```python
from build123d import *

# Parameters (mm, degrees)
F1_DEPTH = 25
F0_W     = 25
F0_H     = 3
F0_H_2   = 15
F2_DEPTH = 3
F3_R     = 2
F4_DEPTH = 25
F3_R_2   = 5
F5_DEPTH = 10


with BuildPart() as f1:
    # F0 (on Top) → F1 (new body)
    with BuildSketch(Plane.XY):
        with BuildLine():
            ThreePointArc((-51.955607151, 33.064927277), (-39.2002565409, 19.8557934078), (-21.4914605021, 15))
            Line((-21.4914605021, 15), (3.5085394979, 15))
            ThreePointArc((3.5085394979, 15), (21.2173355366, 19.8557934078), (33.9726861467, 33.064927277))
            Line((33.9726861467, 33.064927277), (31.3403677316, 34.5039893887))
            ThreePointArc((31.3403677316, 34.5039893887), (19.687169914, 22.4362184053), (3.5085394979, 18))
            Line((3.5085394979, 18), (-21.4914605021, 18))
            ThreePointArc((-21.4914605021, 18), (-37.6700909183, 22.4362184053), (-49.3232887359, 34.5039893887))
            Line((-49.3232887359, 34.5039893887), (-51.955607151, 33.064927277))
        make_face()
    extrude(amount=F1_DEPTH)



with BuildPart() as f1b:
    # F0 (on Top) → F1, piece 2 (new body)
    with BuildSketch(Plane.XY):
        with Locations((-8.9914605021, -1.5)):
            Rectangle(F0_W, F0_H)
    extrude(amount=F1_DEPTH)


with BuildPart() as f1_1:
    add(f1.part)

    add(f1b.part)  # F2 merges F1b
    # F0 (on Top) → F2 (join)
    with BuildSketch(Plane.XY):
        with Locations((-8.9914605021, 7.5)):
            Rectangle(F0_W, F0_H_2)
    extrude(amount=F2_DEPTH)

    # F3 (on face) → F4 (cut)
    with BuildSketch(Plane(origin=(0, 18, 0), x_dir=(-1, 0, 0), z_dir=(0, 1, 0))):
        with Locations((15.4914605021, 12.5)):
            Circle(F3_R)
        with Locations((2.4914605021, 12.5)):
            Circle(F3_R)
    extrude(amount=-F4_DEPTH, mode=Mode.SUBTRACT)

    # F3 (on face) → F5 (cut)
    with BuildSketch(Plane(origin=(0, 18, 0), x_dir=(-1, 0, 0), z_dir=(0, 1, 0))):
        with Locations((15.4914605021, 12.5)):
            Circle(F3_R_2)
        with Locations((15.4914605021, 12.5)):
            Circle(F3_R, mode=Mode.SUBTRACT)
        with Locations((2.4914605021, 12.5)):
            Circle(F3_R_2)
        with Locations((2.4914605021, 12.5)):
            Circle(F3_R, mode=Mode.SUBTRACT)
    extrude(amount=-F5_DEPTH, mode=Mode.SUBTRACT)


solid = f1_1.part
```
The model under review builds one solid part; all positions refer to its coordinate system, in mm. A direction names the side the tool comes from. Coordinates: 2 decimals unless noted, no trailing zeros. Write each loop counter-clockwise with the first axis right and the second up, starting at its lowest first coordinate (ties: lowest second). Pieces come first, ordered by that corner, then holes. Notation, with made-up numbers: (68.5, 12) - (74.5, 12) arc R17 cw to (74.5, 16) - close; hole circle Ø9 at (69, -28). An arc over 180 degrees is marked (long way). Write item = value, one per line.
(1) Consider section C-C, the plane z = 19.25. Give the boundary of the cut face in (x, y).
Result sheet:
outline = (-51.96, 33.06) arc R34.72 ccw to (-21.49, 15) - (3.51, 15) arc R34.72 ccw to (33.97, 33.06) - (31.34, 34.5) arc R31.72 cw to (3.51, 18) - (-21.49, 18) arc R31.72 cw to (-49.32, 34.5) - close; (-21.49, -3) - (3.51, -3) - (3.51, 0) - (-21.49, 0) - close
(2) Machinability: for faces 1 (the face through (-21.491, -1, 9)), 2 (the face through (-9, 15, 14)), 3 (the face through (3.509, -1, 9)), 4 (the face through (-37.47, 22.32, 12.32)), 5 (the face through (-10.496, 16.521, 12.72)), which of the approach directions +Z, -Z, +X, -X, +Y, -Y give a long, thin tool a straight path to every point of the face, cutting with its end or side? Answer none if there is none.
Result sheet:
face_1 = +Z, -Z, -X, -Y
face_2 = +Z, +X, -X
face_3 = +Z, -Z, +X, -Y
face_4 = +Z, -Z, +Y
face_5 = +Y
(3) Consider section D-D, the plane y = 30.5. Give the boundary of the cut face in (x, z).
Result sheet:
outline = (-50.41, 0) - (-46.73, 0) - (-46.73, 25) - (-50.41, 25) - close; (28.74, 0) - (32.42, 0) - (32.42, 25) - (28.74, 25) - close
(4) Consider section B-B, the plane x = -6.5. Give the boundary of the cut face in (y, z), then the cut area to 3 significant figures.
Result sheet:
outline = (-3, 0) - (18, 0) - (18, 9.51) - (15, 9.51) - (15, 3) - (0, 3) - (0, 25) - (-3, 25) - close; (15, 15.49) - (18, 15.49) - (18, 25) - (15, 25) - close
area = 177 mm^2
(5) For line 1 (Y direction, x = -10, z = 3.5); line 2 (Z direction, x = -5.5, y = 17.5); line 3 (X direction, y = 24.5, z = 22.25), list the stretches that pass through material, from the lowest coordinate up. Write a range as [from, to].
Result sheet:
line_1 = [-3, 0], [15, 18]
line_2 = [0, 8.51], [16.49, 25]
line_3 = [-45.35, -40.73], [22.75, 27.37]
(6) Consider section A-A, the plane z = 12.5. Give the boundary of the cut face in (x, y), then the cut area to 3 significant figures.
Result sheet:
outline = (-51.96, 33.06) arc R34.72 ccw to (-21.49, 15) - (-20.49, 15) - (-20.49, 18) - (-21.49, 18) arc R31.72 cw to (-49.32, 34.5) - close; (-21.49, -3) - (-17.49, -3) - (-17.49, 0) - (-21.49, 0) - close; (-13.49, -3) - (-4.49, -3) - (-4.49, 0) - (-13.49, 0) - close; (-10.49, 15) - (-7.49, 15) - (-7.49, 18) - (-10.49, 18) - close; (-0.49, -3) - (3.51, -3) - (3.51, 0) - (-0.49, 0) - close; (2.51, 15) - (3.51, 15) arc R34.72 ccw to (33.97, 33.06) - (31.34, 34.5) arc R31.72 cw to (3.51, 18) - (2.51, 18) - close
area = 279 mm^2
(7) Mouldability with a two-part tool opening along X and no side actions: class faces 6 (the face through (-9, 18, 12)), 7 (the face through (-50.621, 33.795, 12.325)), 8 (the face through (-9, 17, 25)), 9 (the face through (-16.567, -1.479, 14.186)) as pulls with the +X half, pulls with the -X half, needs draft (parallel to the pull), parting line crosses it, or undercut.
Result sheet:
face_6 = undercut
face_7 = pulls with the -X half
face_8 = needs draft
face_9 = undercut
(8) For P1, Ø5, axis at x = -21, z = 22, coming from the +Y side; P2, Ø3.5, axis at x = -2.49, z = 12.5, coming from the -Y side; P3, Ø11, axis at x = -8.5, z = 12.5, coming from the +Y side; P4, Ø14.5, axis at y = 3.5, z = 12, coming from the +X side, all flat-tipped, find the tip position at first contact; note any pin that passes through.
Result sheet:
P1 = 18.06
P2 = through
P3 = 18
P4 = 3.51
